Verification items for the finished model (mm, model axes). Face numbers are marked on the shaded views. Give positions to 0.01 mm unless a question says otherwise; leave off trailing zeros. Write each loop counter-clockwise with the first axis right and the second up, starting at its lowest first coordinate (ties: lowest second). Pieces come first, ordered by that corner, then holes.
from build123d import *

# Parameters (mm, degrees)
PAD_DEPTH    = 1.6
SKETCH001_R  = 1.125
POCKET_DEPTH = 1.601


with BuildPart() as part:
    # Sketch → Pad (new body)
    with BuildSketch(Plane.XY):
        with BuildLine():
            Line((-10, 10), (-2.5, 10))
            ThreePointArc((-2.5, 10), (0, 7.5), (2.5, 10))
            Line((2.5, 10), (10, 10))
            Line((10, 10), (10, 2))
            ThreePointArc((10, -2), (12, 0), (10, 2))
            Line((10, -2), (10, -10))
            Line((10, -10), (2.5, -10))
            ThreePointArc((2.5, -10), (0, -7.5), (-2.5, -10))
            Line((-2.5, -10), (-10, -10))
            Line((-10, -10), (-10, -2))
            ThreePointArc((-10, 2), (-12, 0), (-10, -2))
            Line((-10, 10), (-10, 2))
        make_face()
    extrude(amount=PAD_DEPTH)

    # Sketch001 → Pocket (cut, through all)
    with BuildSketch(Plane.XY):
        with Locations((-10, 0)):
            Circle(SKETCH001_R)
        with Locations((10, 0)):
            Circle(SKETCH001_R)
    extrude(amount=POCKET_DEPTH, mode=Mode.SUBTRACT)


solid = part.part
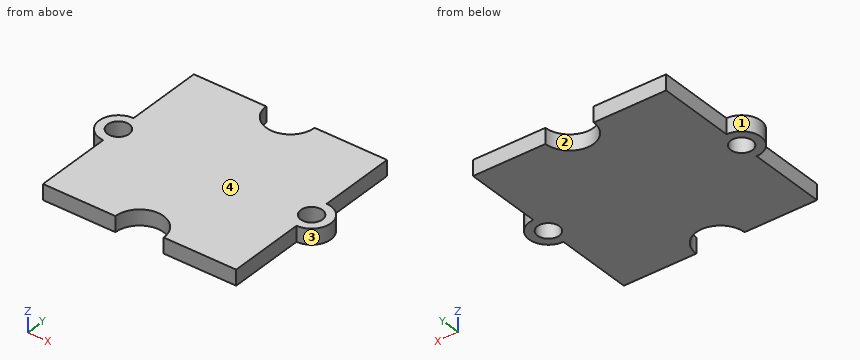
Item 1: Depth check by flat-ended pin: pin 1 (1.3 mm diameter, centred on x = 10, y = 0, fed in from +Z) (3 decimals); pin 2 (0.8 mm diameter, centred on y = -4.5, z = 1, fed in from -X); pin 3 (0.5 mm diameter, centred on y = -4.5, z = 1, fed in from +X). Enter the tip coordinate at first touch or a pass-through.
Answer key:
pin 1: passes through
pin 2: stops at x = -10
pin 3: stops at x = 10
Item 2: Release check for a two-part mould opening along X. For the marked faces 1, 2, 3 and 4 record: released by +X, released by -X, zero draft, split by the parting line, or undercut.
Answer key:
face 1: released by -X
face 2: undercut
face 3: released by +X
face 4: zero draft
Item 3: Sectioned sample at A-A on y = 0. Record the cut outline in (x, z) (3 decimals), then the cut area to 3 significant figures.
Answer key:
outline: (-12, 0) - (-11.125, 0) - (-11.125, 1.6) - (-12, 1.6) - close; (-8.875, 0) - (8.875, 0) - (8.875, 1.6) - (-8.875, 1.6) - close; (11.125, 0) - (12, 0) - (12, 1.6) - (11.125, 1.6) - close
area: 31.2 mm2
Item 4: Scan lines: line 1 along X through (y, z) = (0, 0.4) (3 decimals); line 2 along X through (y, z) = (4.5, 0.35); line 3 along Y through (x, z) = (9.5, 1.55). Record each from-to range of solid material in increasing order.
Answer key:
line 1: x = -12 to -11.125, -8.875 to 8.875, 11.125 to 12
line 2: x = -10 to 10
line 3: y = -10 to -1.01, 1.01 to 10
Item 5: Sectioned sample at B-B on z = 0.9. Record the cut outline in (x, y) (3 decimals), then the cut area to 3 significant figures.
Answer key:
outline: (-10, -10) - (-2.5, -10) arc R2.5 cw to (2.5, -10) - (10, -10) - (10, -2) arc R2 ccw to (10, 2) - (10, 10) - (2.5, 10) arc R2.5 cw to (-2.5, 10) - (-10, 10) - (-10, 2) arc R2 ccw to (-10, -2) - close; hole circle Ø2.25 at (-10, 0); hole circle Ø2.25 at (10, 0)
area: 385 mm2
Item 6: Sectioned sample at C-C on x = -10.5. Record the cut outline in (y, z).
Answer key:
outline: (-1.94, 0) - (-1.01, 0) - (-1.01, 1.6) - (-1.94, 1.6) - close; (1.01, 0) - (1.94, 0) - (1.94, 1.6) - (1.01, 1.6) - close
Item 7: Sectioned sample at D-D on y = 2.75. Record the cut outline in (x, z).
Answer key:
outline: (-10, 0) - (10, 0) - (10, 1.6) - (-10, 1.6) - close
